Could you check a few things on this drawing? It's one solid part, dimensions in mm from its lowest x, y, z. A direction names the side the tool comes from. Round coordinates to 2 decimals unless told otherwise and drop trailing zeros. Loops run counter-clockwise (first coordinate to the right, second up) from the corner with the lowest first, then second, coordinate; pieces in that order, holes last. Notation, with made-up numbers: M 1,-21.5 L 6,-21.5 A28 ccw 6,10.5 Z; hole C 48,45.25 d7. An arc over 180 degrees is marked long. Use a Markdown table: item, result. Add a question column.
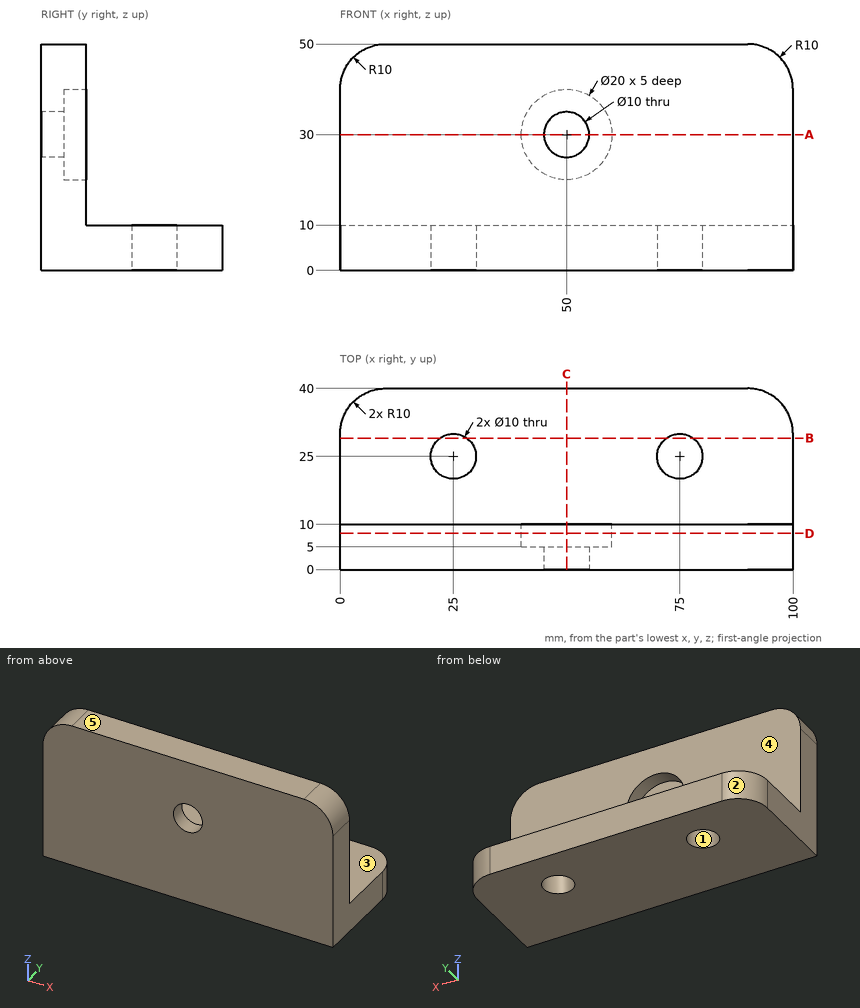
(1) Suppose I cut it at C-C on x = 50. List the corners of the cut face in (y, z) for me, and give its area (3 significant figures).
(2) Suppose I cut it at B-B on y = 29. List the corners of the cut face in (x, z) for me.
(3) Thinking about a two-plate mould opening in X: for the marked faces 1, 2 and 3, which applies, released by +X, released by -X, zero draft, split by the parting line, or undercut?
(4) I'm going to push flat-ended pins straight in: pin 1 (10 mm diameter, centred on x = 56, z = 23, fed in from +Y); pin 2 (15 mm diameter, centred on x = 60, y = 23, fed in from +Z); pin 3 (6 mm diameter, centred on x = 53, z = 26.5, fed in from +Y); pin 4 (8 mm diameter, centred on x = 25, y = 25, fed in from -Z). Where does each tip first touch, or does it pass through?
(5) If I drill on probe 1 along Y at (x, z) = (75, 5); probe 2 along Z at (x, y) = (50, 7); probe 3 along Z at (x, y) = (50, 1.7), over which ranges is the centre line in solid material (lowest first)? Write a range as [from, to].
(6) Suppose I cut it at D-D on y = 8. List the corners of the cut face in (x, z) for me, and give its area (3 significant figures).
(7) Suppose I cut it at A-A on z = 30. List the corners of the cut face in (x, y) for me.
(8) On a 3-axis mill with a long thin cutter (end or side, diameter ignored), from which of +Z, -Z, +X, -X, +Y, -Y can I reach the whole of each face in a straight line? I mean the marked faces 4 and 5. Say none if no direction works.
Results below:
| question | item | result |
|---|---|---|
| 1 | outline | M 0,0 L 40,0 L 40,10 L 10,10 L 10,20 L 5,20 L 5,25 L 0,25 Z; M 0,35 L 5,35 L 5,40 L 10,40 L 10,50 L 0,50 Z |
| 1 | area | 650 mm² |
| 2 | outline | M 0,0 L 22,0 L 22,10 L 0,10 Z; M 28,0 L 72,0 L 72,10 L 28,10 Z; M 78,0 L 100,0 L 100,10 L 78,10 Z |
| 3 | face 1 | undercut |
| 3 | face 2 | released by -X |
| 3 | face 3 | zero draft |
| 4 | pin 1 | stops at y = 10 |
| 4 | pin 2 | stops at z = 10 |
| 4 | pin 3 | stops at y = 5 |
| 4 | pin 4 | passes through |
| 5 | probe 1 | y = [0, 20], [30, 40] |
| 5 | probe 2 | z = [0, 20], [40, 50] |
| 5 | probe 3 | z = [0, 25], [35, 50] |
| 6 | outline | M 0,0 L 100,0 L 100,40 A10 ccw 90,50 L 10,50 A10 ccw 0,40 Z; hole C 50,30 d20 |
| 6 | area | 4,640 mm² |
| 7 | outline | M 0,0 L 45,0 L 45,5 L 40,5 L 40,10 L 0,10 Z; M 55,0 L 100,0 L 100,10 L 60,10 L 60,5 L 55,5 Z |
| 8 | face 4 | +Z, +X, -X, +Y |
| 8 | face 5 | +Z, +X, -X, +Y, -Y |
